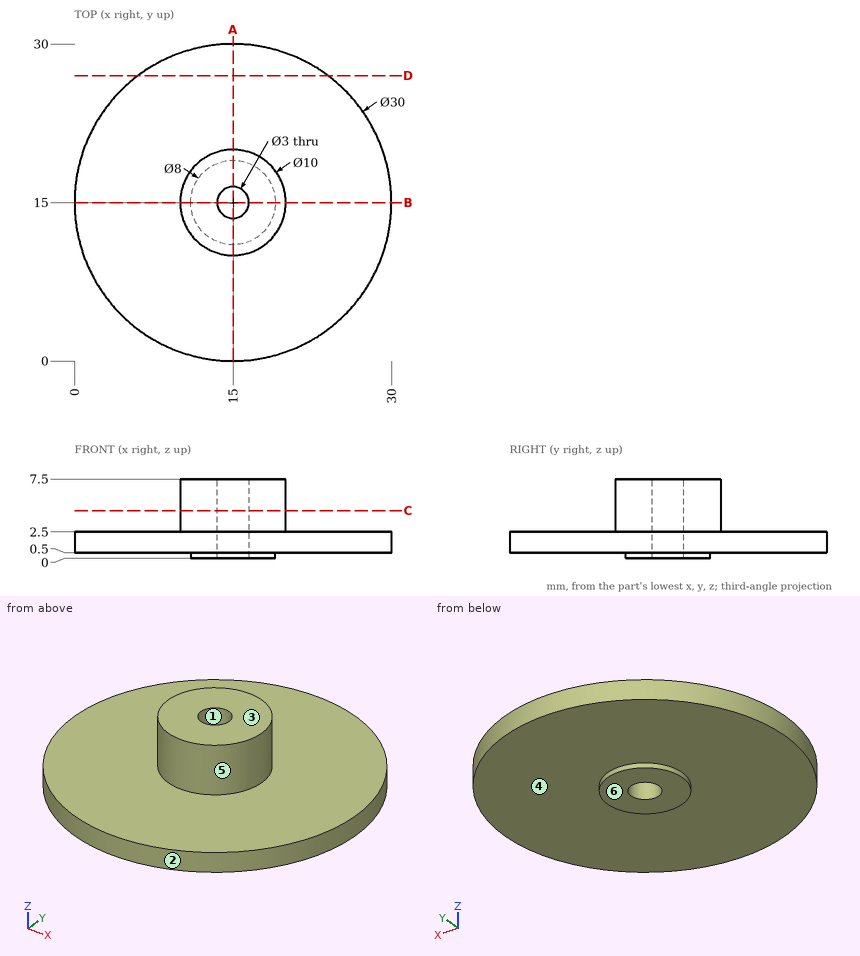
For this review, use the dimensioned drawing (mm, ordinates from the lowest corner) and the shaded views. A direction names the side the tool comes from. Coordinates: 2 decimals unless noted, no trailing zeros. Order: outer loops, then holes, each group sorted by start corner. A loop starts at its lowest first (then second) coordinate and runs counter-clockwise, first axis right, second up. Notation, with made-up numbers: (-39, 35) - (-12, 35) arc R13 ccw to (-12, 44) - close; hole circle Ø1 at (17, 73.5). An arc over 180 degrees is marked (long way). Answer in a Markdown table with one row per item.
(1) Consider section D-D on y = 27. State the section outline as (x, z) points.
Checked values:
| item | result |
|---|---|
| outline | (6, 0.5) - (24, 0.5) - (24, 2.5) - (6, 2.5) - close |
(2) Clearance check with flat-ended pins moving along their axes: pin 1 (4 mm diameter, centred on x = 17.5, z = 2, fed in from +Y); pin 2 (4 mm diameter, centred on x = 5, y = 13.5, fed in from -Z); pin 3 (3 mm diameter, centred on y = 24.5, z = 2, fed in from +X). State where each tip first meets the part, or that it passes through.
Checked values:
| item | result |
|---|---|
| pin 1 | y = 29.99 |
| pin 2 | z = 0.5 |
| pin 3 | x = 27.69 |
(3) Wall thickness on line 1 along Y through (x, z) = (15, 5.5); line 2 along Z through (x, y) = (9.75, 4.75); line 3 along Y through (x, z) = (14.5, 4.5): over which ranges is each line inside the solid? List them lowest first. Write a range as from..to.
Checked values:
| item | result |
|---|---|
| line 1 | 10..13.5, 16.5..20 |
| line 2 | 0.5..2.5 |
| line 3 | 10.03..13.59, 16.41..19.97 |
(4) Consider section A-A on x = 15. State the section outline as (y, z) points.
Checked values:
| item | result |
|---|---|
| outline | (0, 0.5) - (11, 0.5) - (11, 0) - (13.5, 0) - (13.5, 7.5) - (10, 7.5) - (10, 2.5) - (0, 2.5) - close; (16.5, 0) - (19, 0) - (19, 0.5) - (30, 0.5) - (30, 2.5) - (20, 2.5) - (20, 7.5) - (16.5, 7.5) - close |
(5) The part is to be moulded in two halves that separate along X. For the marked faces 1, 2 and 3, say which applies: released by +X, released by -X, zero draft, split by the parting line, or undercut.
Checked values:
| item | result |
|---|---|
| face 1 | undercut |
| face 2 | split by the parting line |
| face 3 | zero draft |
(6) Consider section C-C on z = 4.5. State the section outline as (x, y) points.
Checked values:
| item | result |
|---|---|
| outline | circle Ø10 at (15, 15); hole circle Ø3 at (15, 15) |
(7) For the marked faces 4, 5 and 6, list the 3-axis set-ups (+Z, -Z, +X, -X, +Y, -Y) from which the entire face can be reached by the end or side of a thin tool; tool diameter is ignored.
Checked values:
| item | result |
|---|---|
| face 4 | -Z |
| face 5 | +Z |
| face 6 | -Z, +X, -X, +Y, -Y |
